Verification items for the finished model (mm, model axes). A direction names the side the tool comes from. Round coordinates to 2 decimals unless told otherwise and drop trailing zeros. Write each loop counter-clockwise with the first axis right and the second up, starting at its lowest first coordinate (ties: lowest second). Pieces come first, ordered by that corner, then holes. Notation, with made-up numbers: M 28,-11.5 L 55,-11.5 A10 cw 55,6.5 Z; hole C 0,2 d5. An arc over 180 degrees is marked long. One line per item, written item: value. Start each with the question number.
Item 1: Tool access check on faces 1 (the face through (-25.4, 82, 4)), 2 (the face through (20, 44.45, -12)), 3 (the face through (25, 59, -15.875)), 4 (the face through (20, 44.45, 12)). Record the directions out of +Z, -Z, +X, -X, +Y, -Y that give a thin tool (end or side, any length) a straight path to the whole face; none if there is none.
Item 2: Thickness scan on probe 1 along X at (y, z) = (8, 0) (3 decimals); probe 2 along X at (y, z) = (88.5, 11.5); probe 3 along Z at (x, y) = (-28, 55.5) (3 decimals). Record the ranges inside material, lowest first. Write a range as from..to.
Item 3: Gauge pin test, flat ends, axial feed: pin 1 (1 mm diameter, centred on x = 5.5, z = -11.5, fed in from -Y); pin 2 (8 mm diameter, centred on y = 18, z = -15.5, fed in from +X); pin 3 (8 mm diameter, centred on x = 26, y = 71, fed in from -Z) (3 decimals). Record the tip position at first contact, or that the pin passes through.
Item 4: Section check D-D, the plane x = 27.5. Record the cut outline in (y, z) (3 decimals).
Item 5: Draft check along Y on faces 5 (the face through (-15.1, 0, -5.4)), 6 (the face through (-28.531, 91.628, 12.056)), 7 (the face through (28.53, 70, -1.38)). Enter one of: +Y half, -Y half, draft (parallel to the pull), parting line (faces both ways), or undercut.
Item 6: Section check A-A, the plane y = 64.5. Record the cut outline in (x, z) (3 decimals), then the cut area to 3 significant figures.
Item 7: Section check C-C, the plane x = -4. Record the cut outline in (y, z) (3 decimals), then the cut area to 3 significant figures.
Item 8: Section check B-B, the plane y = 76.2. Record the cut outline in (x, z) (3 decimals).
from build123d import *

# Parameters (mm, degrees)
SKETCH2_R           = 18.415
SKETCH2_R_2         = 15.875
BOSS_EXTRUDE1_DEPTH = 38.1
SKETCH3_R           = 22.225
BOSS_EXTRUDE2_DEPTH = 6.35
SKETCH5_W           = 63.5
SKETCH5_H           = 31.75
BOSS_EXTRUDE3_DEPTH = 50.8
CUT_EXTRUDE2_DEPTH  = 50.8
FILLET1_R           = 12.7
SKETCH9_R           = 6.35
CUT_EXTRUDE3_DEPTH  = 117.613734719
FILLET2_R           = 12.7


with BuildPart() as part:
    # Sketch2 → Boss-Extrude1 (new body)
    with BuildSketch(Plane(origin=(0, 0, 0), x_dir=(1, 0, 0), z_dir=(0, 1, 0))):
        with Locations(Location((0, 0, 0), (0, 0, 90))):
            Circle(SKETCH2_R)
        with Locations(Location((0, 0, 0), (0, 0, 90))):
            Circle(SKETCH2_R_2, mode=Mode.SUBTRACT)
    extrude(amount=BOSS_EXTRUDE1_DEPTH)

    # Sketch3 → Boss-Extrude2 (add)
    with BuildSketch(Plane(origin=(0, 38.1, 0), x_dir=(1, 0, 0), z_dir=(0, 1, 0))):
        with Locations(Location((0, 0, 0), (0, 0, 270))):
            Circle(SKETCH3_R)
    extrude(amount=BOSS_EXTRUDE2_DEPTH)

    # Sketch5 → Boss-Extrude3 (add)
    with BuildSketch(Plane(origin=(0, 44.45, 0), x_dir=(1, 0, 0), z_dir=(0, 1, 0))):
        Rectangle(SKETCH5_W, SKETCH5_H)
    extrude(amount=BOSS_EXTRUDE3_DEPTH)

    # Sketch7 → Cut-Extrude2 (cut)
    with BuildSketch(Plane.XY.offset(15.875)):
        Polygon((25.4, 95.25), (-25.4, 95.25), (-25.4, 60.667652482), (-15.532347518, 50.8), (15.532347518, 50.8), (25.4, 60.667652482), align=None)
        Polygon((-22.225, 44.45), (-31.75, 53.975), (-31.75, 44.45), align=None)
        Polygon((22.225, 44.45), (31.75, 53.975), (31.75, 44.45), align=None)
    extrude(amount=-CUT_EXTRUDE2_DEPTH, mode=Mode.SUBTRACT)

    # Fillet1
    fillet1_edges = [part.edges().sort_by_distance(p)[0] for p in [
        (28.575, 95.25, -15.875),
        (-28.575, 95.25, 15.875),
        (-28.575, 95.25, -15.875),
        (28.575, 95.25, 15.875),
    ]]
    fillet(fillet1_edges, radius=FILLET1_R)

    # Sketch9 → Cut-Extrude3 (cut, through all)
    with BuildSketch(Plane.ZY.offset(31.75)):
        with Locations((0, 76.2)):
            Circle(SKETCH9_R)
    extrude(amount=-CUT_EXTRUDE3_DEPTH, mode=Mode.SUBTRACT)

    # Fillet2
    # the kernel refuses this fillet: 12.7 mm, written as the material it adds along each edge
    with BuildSketch(Plane(origin=(-43.050566437, 44.45, 15.875), x_dir=(0, 1, 0), z_dir=(1, 0, 0))) as fillet2_piece_1_section:
        with BuildLine():
            CenterArc((12.7, 10.998522628), FILLET2_R, 180, 60)
            Line((0, 10.998522628), (0, 0))
            Line((0, 0), (6.35, 0))
        make_face()
    fillet2_piece_1 = extrude(amount=86.101132874, mode=Mode.PRIVATE)
    fillet2_piece_1 = fillet2_piece_1 & Plane(origin=(0, 49.09130813, 0), x_dir=(0, 0, 1), z_dir=(0, -1, 0)) * Cylinder(22.225, 217, mode=Mode.PRIVATE)
    add(fillet2_piece_1)
    with BuildSketch(Plane(origin=(43.050566437, 44.45, -15.875), x_dir=(0, 1, 0), z_dir=(-1, 0, 0))) as fillet2_piece_2_section:
        with BuildLine():
            CenterArc((12.7, 10.998522628), FILLET2_R, 180, 60)
            Line((0, 10.998522628), (0, 0))
            Line((0, 0), (6.35, 0))
        make_face()
    fillet2_piece_2 = extrude(amount=86.101132874, mode=Mode.PRIVATE)
    fillet2_piece_2 = fillet2_piece_2 & Plane(origin=(0, 49.09130813, 0), x_dir=(0, 0, 1), z_dir=(0, -1, 0)) * Cylinder(22.225, 217, mode=Mode.PRIVATE)
    add(fillet2_piece_2)


solid = part.part
Response values:
1. face 1: +Z, -Z, +Y
1. face 2: -Z, +X, -Y
1. face 3: -Z, +X, +Y, -Y
1. face 4: +Z, +X, -Y
2. probe 1: x = -18.415..-15.875, 15.875..18.415
2. probe 2: x = -31.75..-25.4, 25.4..31.75
2. probe 3: z = -15.875..15.875
3. pin 1: stops at y = 38.1
3. pin 2: stops at x = 14.38
3. pin 3: stops at z = -15.875
4. outline: M 49.725,-15.875 L 82.55,-15.875 A12.7 ccw 95.25,-3.175 L 95.25,3.175 A12.7 ccw 82.55,15.875 L 49.725,15.875 Z; hole C 76.2,0 d12.7
5. face 5: -Y half
5. face 6: +Y half
5. face 7: undercut
6. outline: M -31.75,-15.875 L -25.4,-15.875 L -25.4,15.875 L -31.75,15.875 Z; M 25.4,-15.875 L 31.75,-15.875 L 31.75,15.875 L 25.4,15.875 Z
6. area: 403 mm2
7. outline: M 0,-17.975 L 38.1,-17.975 L 38.1,-21.862 L 45.481,-21.862 A12.7 cw 50.8,-15.875 L 50.8,15.875 A12.7 cw 45.481,21.862 L 38.1,21.862 L 38.1,17.975 L 0,17.975 L 0,15.363 L 38.1,15.363 L 38.1,-15.363 L 0,-15.363 Z
7. area: 716 mm2
8. outline: M -31.75,-15.875 L -25.4,-15.875 L -25.4,-6.35 L -31.75,-6.35 Z; M -31.75,6.35 L -25.4,6.35 L -25.4,15.875 L -31.75,15.875 Z; M 25.4,-15.875 L 31.75,-15.875 L 31.75,-6.35 L 25.4,-6.35 Z; M 25.4,6.35 L 31.75,6.35 L 31.75,15.875 L 25.4,15.875 Z
